Geometry check sheet. Reference: drawing and pictorial views, mm from the part's lowest x, y, z. A direction names the side the tool comes from. Coordinates: 2 decimals unless noted, no trailing zeros. Write each loop counter-clockwise with the first axis right and the second up, starting at its lowest first coordinate (ties: lowest second). Pieces come first, ordered by that corner, then holes. Notation, with made-up numbers: (61, -33) -> (94, -33) arc R11 ccw to (94, -24) -> close; hole circle Ø8 at (-30.5, -26). An arc over 180 degrees is marked (long way). Answer in a Markdown table with one row per item.
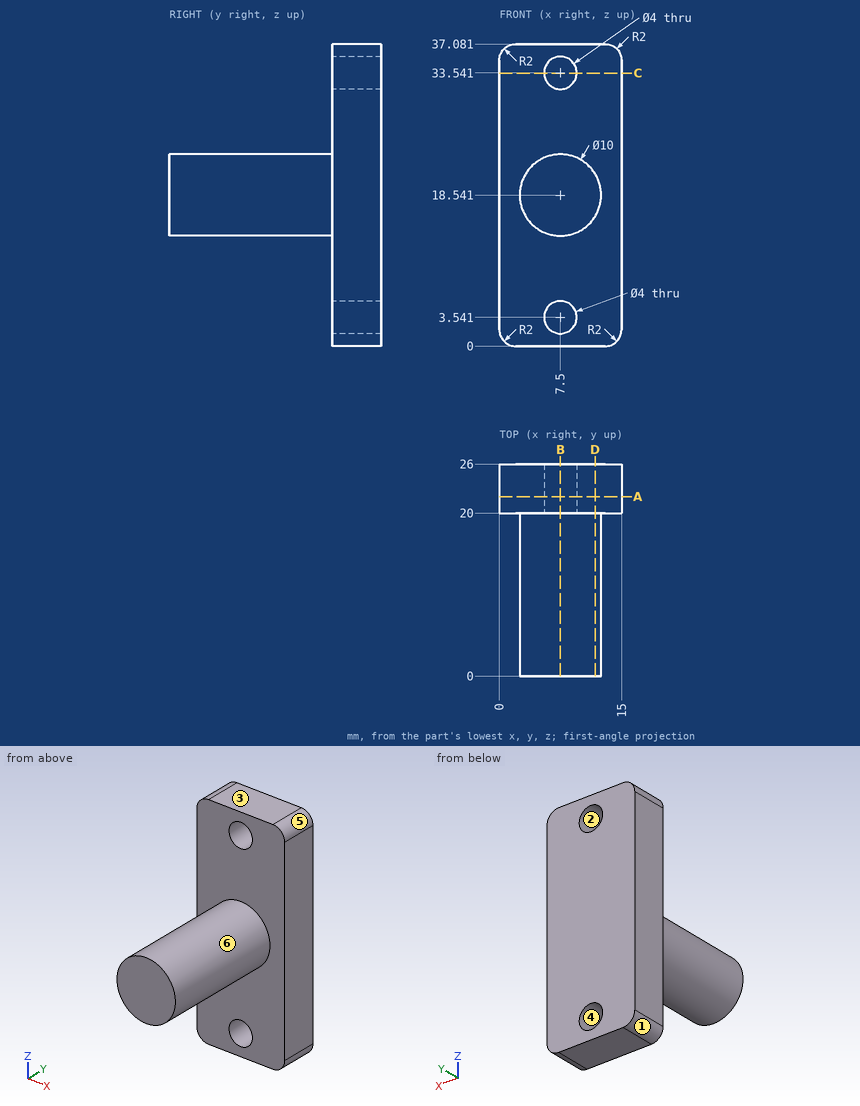
1. Mould release check, pull along X, two halves, no side actions. Record for the marked faces 1, 2, 3 and 4: released by +X, released by -X, zero draft, split by the parting line, or undercut.
Geometry says:
| item | result |
|---|---|
| face 1 | released by -X |
| face 2 | undercut |
| face 3 | zero draft |
| face 4 | undercut |
2. Section check D-D, the plane x = 11.75. Record the boundary of the cut face in (y, z) (1 decimal).
Geometry says:
| item | result |
|---|---|
| outline | (0, 15.9) -> (20, 15.9) -> (20, 0) -> (26, 0) -> (26, 37.1) -> (20, 37.1) -> (20, 21.2) -> (0, 21.2) -> close |
3. Section check A-A, the plane y = 22. Record the boundary of the cut face in (x, z), plus the area to 3 significant figures.
Geometry says:
| item | result |
|---|---|
| outline | (0, 2) arc R2 ccw to (2, 0) -> (13, 0) arc R2 ccw to (15, 2) -> (15, 35.08) arc R2 ccw to (13, 37.08) -> (2, 37.08) arc R2 ccw to (0, 35.08) -> close; hole circle Ø4 at (7.5, 3.54); hole circle Ø4 at (7.5, 33.54) |
| area | 528 mm^2 |
4. Thickness scan on line 1 (Z direction, x = 7.5, y = 20.5); line 2 (Z direction, x = 7.5, y = 15); line 3 (Y direction, x = 4.25, z = 23.5). Record the ranges inside material, lowest first. Write a range as from..to.
Geometry says:
| item | result |
|---|---|
| line 1 | 0..1.54, 5.54..31.54, 35.54..37.08 |
| line 2 | 13.54..23.54 |
| line 3 | 20..26 |
5. Depth check by flat-ended pin: P1, Ø2.5, axis at x = 7.5, z = 3.54, coming from the -Y side; P2, Ø8, axis at y = 10, z = 12, coming from the -X side; P3, Ø2, axis at y = 9.5, z = 13.5, coming from the -X side (1 decimal); P4, Ø2, axis at y = 14, z = 23, coming from the -X side. Enter the tip coordinate at first touch or a pass-through.
Geometry says:
| item | result |
|---|---|
| P1 | through |
| P2 | x = 3.19 |
| P3 | x = 4.6 |
| P4 | x = 3.89 |
6. Section check B-B, the plane x = 7.5. Record the boundary of the cut face in (y, z).
Geometry says:
| item | result |
|---|---|
| outline | (0, 13.54) -> (20, 13.54) -> (20, 5.54) -> (26, 5.54) -> (26, 31.54) -> (20, 31.54) -> (20, 23.54) -> (0, 23.54) -> close; (20, 0) -> (26, 0) -> (26, 1.54) -> (20, 1.54) -> close; (20, 35.54) -> (26, 35.54) -> (26, 37.08) -> (20, 37.08) -> close |
7. Section check C-C, the plane z = 33.5. Record the boundary of the cut face in (x, y).
Geometry says:
| item | result |
|---|---|
| outline | (0, 20) -> (5.5, 20) -> (5.5, 26) -> (0, 26) -> close; (9.5, 20) -> (15, 20) -> (15, 26) -> (9.5, 26) -> close |
8. Tool access check on the marked faces 5 and 6. Record the directions out of +Z, -Z, +X, -X, +Y, -Y that give a thin tool (end or side, any length) a straight path to the whole face; none if there is none.
Geometry says:
| item | result |
|---|---|
| face 5 | +Z, +X, +Y, -Y |
| face 6 | -Y |
